Source: CAD feature listing. Evaluate the final solid. Frame: model axes, mm. A direction names the side the tool comes from. Give positions to 0.01 mm unless a question says otherwise; leave off trailing zeros. Order: outer loops, then holes, each group sorted by start corner. A loop starts at its lowest first (then second) coordinate and runs counter-clockwise, first axis right, second up. Notation, with made-up numbers: M 79.25,11.25 L 104.25,11.25 A28 cw 104.25,49.25 Z; hole C 67,51.25 d11. An arc over 180 degrees is marked long. Answer as a JSON object with one key per item and string values. Group by question number.
1. Set-up query: faces 1 (the cylindrical face through (-3.233, 1.341, 2.024)), 2 (the cylindrical face through (0, -2, -4)), 3 (the flat face through (-1.3, -0.74, 2.52)). Return all of +Z, -Z, +X, -X, +Y, -Y with unobstructed straight access to the full face (end or side cutting, diameter ignored); none if empty.
2. Pin query (flat end, axial travel): P1, Ø3.5, axis at x = 1, y = 0, coming from the +Z side; P2, Ø2, axis at y = -1, z = -4.5, coming from the +X side; P3, Ø4, axis at x = -2, z = -2.5, coming from the +Y side; P4, Ø1.5, axis at x = 0, y = -0.5, coming from the +Z side. Return the tip coordinate at first contact, or that it passes through.
3. Material intervals for L1, parallel to Z at x = 2, y = -1.5; L2, parallel to Z at x = 1.25, y = -0.5; L3, parallel to X at y = -1, z = 2.75, sorted ascending. Write a range as [from, to].
4. Section query A-A (z = 2.5). Output: boundary loops of the cut face in (x, y), plus the area to 3 significant figures.
5. Section query B-B (x = 0). Output: boundary loops of the cut face in (y, z), plus the area to 3 significant figures.
6. Section query C-C (z = -4). Output: boundary loops of the cut face in (x, y).
from build123d import *

# Parameters (mm, degrees)
SKETCH1_R           = 3.5
BOSS_EXTRUDE1_DEPTH = 4
SKETCH2_R           = 2
BOSS_EXTRUDE2_DEPTH = 8
CUT_EXTRUDE1_DEPTH  = 3
CHAMFER1_SIZE       = 0.25


with BuildPart() as part:
    # Sketch1 → Boss-Extrude1 (new body)
    with BuildSketch(Plane.XY.offset(4)):
        with Locations(Location((0, 0, 0), (0, 0, 180))):
            Circle(SKETCH1_R)
    extrude(amount=-BOSS_EXTRUDE1_DEPTH)

    # Sketch2 → Boss-Extrude2 (add)
    with BuildSketch(Plane(origin=(0, 0, 0), x_dir=(-1, 0, 0), z_dir=(0, 0, -1))):
        Circle(SKETCH2_R)
    extrude(amount=BOSS_EXTRUDE2_DEPTH)

    # Sketch3 → Cut-Extrude1 (cut)
    with BuildSketch(Plane.XY.offset(4)):
        Polygon((-1.726010921, 0), (-0.863005461, -1.494769305), (0.863005461, -1.494769305), (1.726010921, 0), (0.863005461, 1.494769305), (-0.863005461, 1.494769305), align=None)
    extrude(amount=-CUT_EXTRUDE1_DEPTH, mode=Mode.SUBTRACT)

    # Chamfer1
    chamfer1_edges = [part.edges().sort_by_distance(p)[0] for p in [
        (3.5, 0, 4),
        (3.5, 0, 0),
        (2, 0, -8),
    ]]
    chamfer(chamfer1_edges, length=CHAMFER1_SIZE)


solid = part.part
Answer sheet:
{
 "1": {"face 1": "+Z, -Z", "face 2": "-Z", "face 3": "+Z"},
 "2": {"P1": "z = 4", "P2": "x = 2", "P3": "y = 2", "P4": "z = 1"},
 "3": {"L1": "[0, 4]", "L2": "[-8, 1]", "L3": "[-3.35, -1.15], [1.15, 3.35]"},
 "4": {"outline": "C 0,0 d7; hole M -1.73,0 L -0.86,-1.49 L 0.86,-1.49 L 1.73,0 L 0.86,1.49 L -0.86,1.49 Z", "area": "30.7 mm^2"},
 "5": {"outline": "M -3.5,0.25 L -3.25,0 L -2,0 L -2,-7.75 L -1.75,-8 L 1.75,-8 L 2,-7.75 L 2,0 L 3.25,0 L 3.5,0.25 L 3.5,3.75 L 3.25,4 L 1.49,4 L 1.49,1 L -1.49,1 L -1.49,4 L -3.25,4 L -3.5,3.75 Z", "area": "50.8 mm^2"},
 "6": {"outline": "C 0,0 d4"}
}
